```python
from build123d import *

# Parameters (mm, degrees)
BOSS_EXTRUDE2_DEPTH = 22.5
FILLET1_R           = 3
SKETCH2_R           = 3
CUT_EXTRUDE1_DEPTH  = 45
CUT_EXTRUDE2_DEPTH  = 34.768920734


with BuildPart() as part:
    # Sketch1 → Boss-Extrude2 (new, symmetric)
    with BuildSketch(Plane.XY):
        with BuildLine():
            Line((0, 10.65), (0, 20))
            Line((0, 20), (6, 20))
            Line((6, 20), (6, 14.074444927))
            ThreePointArc((6, 14.074444927), (15.3, 0), (6, -14.074444927))
            Line((6, -14.074444927), (6, -20))
            Line((6, -20), (0, -20))
            Line((0, -20), (0, -10.65))
            ThreePointArc((0, -10.65), (10.65, 0), (0, 10.65))
        make_face()
    extrude(amount=BOSS_EXTRUDE2_DEPTH, both=True)

    # Fillet1
    fillet1_edges = [part.edges().sort_by_distance(p)[0] for p in [
        (6, 14.074444927, 0),
        (6, -14.074444927, 0),
    ]]
    fillet(fillet1_edges, radius=FILLET1_R)

    # Sketch2 → Cut-Extrude1 (cut)
    with BuildSketch(Plane.ZY):
        with Locations((-17.8, 15.3)):
            Circle(SKETCH2_R)
        with Locations((17.8, 15.3)):
            Circle(SKETCH2_R)
        with Locations((17.8, -15.3)):
            Circle(SKETCH2_R)
        with Locations((-17.8, -15.3)):
            Circle(SKETCH2_R)
    extrude(amount=-CUT_EXTRUDE1_DEPTH, mode=Mode.SUBTRACT)

    # Sketch3 → Cut-Extrude2 (cut, through all)
    with BuildSketch(Plane.ZY):
        with BuildLine():
            Line((16, 7.5), (10, 7.5))
            ThreePointArc((10, 7.5), (0, 3.297958971), (-10, 7.5))
            Line((-10, 7.5), (-16, 7.5))
            Line((-16, 7.5), (-16, -7.5))
            Line((-16, -7.5), (-10, -7.5))
            ThreePointArc((-10, -7.5), (0, -3.297958971), (10, -7.5))
            Line((10, -7.5), (16, -7.5))
            Line((16, -7.5), (16, 7.5))
        make_face()
    extrude(amount=-CUT_EXTRUDE2_DEPTH, mode=Mode.SUBTRACT)


solid = part.part
```
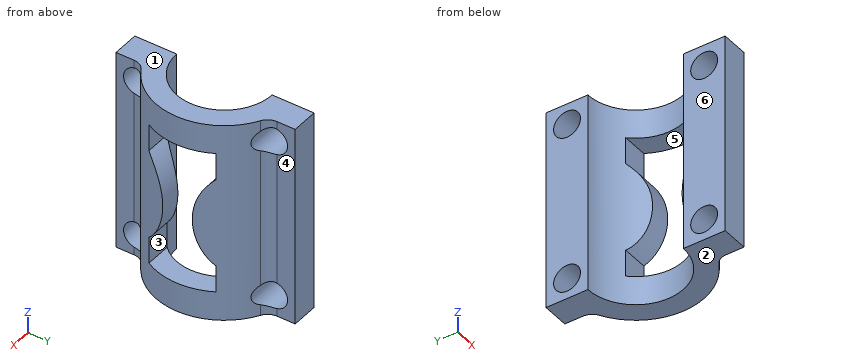
Verification items for the finished model (mm, model axes). Face numbers are marked on the shaded views. A direction names the side the tool comes from. Round coordinates to 2 decimals unless told otherwise and drop trailing zeros. Write each loop counter-clockwise with the first axis right and the second up, starting at its lowest first coordinate (ties: lowest second). Pieces come first, ordered by that corner, then holes. Notation, with made-up numbers: (52.25, 9.25) -> (82.25, 9.25) arc R28 cw to (82.25, 28.25) -> close; hole circle Ø9 at (-24.5, 20). An arc over 180 degrees is marked (long way). Write each question's results on one line, items separated by ' | '.
Q1. Go/stop test with flat-tipped pins: pin 1 Ø1.7 at (x, z) = (9.5, -13.5) entering from +Y; pin 2 Ø4.5 at (y, z) = (17.5, 4) entering from +X; pin 3 Ø3 at (y, z) = (-1, -1) entering from -X; pin 4 Ø8 at (x, y) = (7, -7.5) entering from -Z. Record where each tip stops, or that it passes through.
Derived:
pin 1: stops at y = 12.62 | pin 2: stops at x = 6.08 | pin 3: passes through | pin 4: stops at z = -22.5
Q2. Sectioned sample at B-B, the plane z = 17.8. Record the boundary of the cut face in (x, y), and give its area (3 significant figures).
Derived:
outline: (0, -20) -> (6, -20) -> (6, -18.3) -> (0, -18.3) -> close; (0, -12.3) -> (9.1, -12.3) arc R15.3 ccw to (9.1, 12.3) -> (0, 12.3) -> (0, 10.65) arc R10.65 cw to (0, -10.65) -> close; (0, 18.3) -> (6, 18.3) -> (6, 20) -> (0, 20) -> close | area: 173 mm²
Q3. Sectioned sample at C-C, the plane y = -6. Record the boundary of the cut face in (x, z), and give its area (3 significant figures).
Derived:
outline: (8.8, -22.5) -> (14.07, -22.5) -> (14.07, -16) -> (8.8, -16) -> close; (8.8, -8.27) -> (14.07, -8.27) -> (14.07, 8.27) -> (8.8, 8.27) -> close; (8.8, 16) -> (14.07, 16) -> (14.07, 22.5) -> (8.8, 22.5) -> close | area: 156 mm²
Q4. Sectioned sample at D-D, the plane z = 7.5. Record the boundary of the cut face in (x, y), and give its area (3 significant figures).
Derived:
outline: (0, -20) -> (6, -20) -> (6, -15.93) arc R3 cw to (7.52, -13.32) arc R15.3 ccw to (14.29, -5.48) -> (9.13, -5.48) arc R10.65 cw to (0, -10.65) -> close; (0, 10.65) arc R10.65 cw to (9.13, 5.48) -> (14.29, 5.48) arc R15.3 ccw to (7.52, 13.32) arc R3 cw to (6, 15.93) -> (6, 20) -> (0, 20) -> close | area: 199 mm²
Q5. Thickness scan on probe 1 along Z at (x, y) = (2, 15.3); probe 2 along Z at (x, y) = (12.75, -4.5); probe 3 along Y at (x, z) = (5.5, 18.5). Record the ranges inside material, lowest first.
Derived:
probe 1: z = -22.5 to -20.8, -14.8 to 14.8, 20.8 to 22.5 | probe 2: z = -22.5 to -16, -5.68 to 5.68, 16 to 22.5 | probe 3: y = -20 to -18.22, -12.38 to -9.12, 9.12 to 12.38, 18.22 to 20
Q6. Draft check along Z on the marked faces 1, 2, 3 and 4. Enter one of: released by +Z, released by -Z, zero draft, split by the parting line, or undercut.
Derived:
face 1: released by +Z | face 2: released by -Z | face 3: undercut | face 4: zero draft
Q7. Sectioned sample at A-A, the plane x = 3. Record the boundary of the cut face in (y, z), and give its area (3 significant figures).
Derived:
outline: (-20, -22.5) -> (-10.22, -22.5) -> (-10.22, 22.5) -> (-20, 22.5) -> close; (10.22, -22.5) -> (20, -22.5) -> (20, 22.5) -> (10.22, 22.5) -> close; hole circle Ø6 at (-15.3, -17.8); hole circle Ø6 at (-15.3, 17.8); hole circle Ø6 at (15.3, -17.8); hole circle Ø6 at (15.3, 17.8) | area: 767 mm²
Q8. Access from +Z, -Z, +X, -X, +Y, -Y to the whole of each face (thin tool, end or side, straight path). Record for the marked faces 5 and 6.
Derived:
face 5: +X, -X | face 6: +Z, -Z, -X, +Y, -Y
